```python
from build123d import *

# Parameters (mm, degrees)
F0_R      = 20
F1_DEPTH  = 47.5
F3_DEPTH  = 30
F5_DEPTH  = 25
F7_DEPTH  = 30
F8_R      = 6
F9_DEPTH  = 25
F10_DEPTH = 57.501


with BuildPart() as f1:
    # F0 (on Front) → F1 (new body, symmetric)
    with BuildSketch(Plane.XZ):
        Circle(F0_R)
    extrude(amount=F1_DEPTH, both=True)

    # F2 (on face) → F3 (cut)
    with BuildSketch(Plane.XZ.offset(47.5)):
        with BuildLine():
            ThreePointArc((8, 18.3303027798), (0, 20), (-8, 18.3303027798))
            Line((-8, 18.3303027798), (-8, -18.3303027798))
            ThreePointArc((-8, -18.3303027798), (0, -20), (8, -18.3303027798))
            Line((8, -18.3303027798), (8, 18.3303027798))
        make_face()
    extrude(amount=-F3_DEPTH, mode=Mode.SUBTRACT)

    # F4 (on face) → F5 (cut)
    with BuildSketch(Plane.XZ.offset(47.5)):
        with BuildLine():
            Line((-18, -8.7177978871), (-18, 8.7177978871))
            ThreePointArc((-18, 8.7177978871), (-20, 0), (-18, -8.7177978871))
        make_face()
        with BuildLine():
            ThreePointArc((20, 0), (19.4935886896, 4.472135955), (18, 8.7177978871))
            Line((18, 8.7177978871), (18, -8.7177978871))
            ThreePointArc((18, -8.7177978871), (19.4935886896, -4.472135955), (20, 0))
        make_face()
    extrude(amount=-F5_DEPTH, mode=Mode.SUBTRACT)

    # F6 (on face) → F7 (cut)
    with BuildSketch(Plane(origin=(0, 47.5, 0), x_dir=(-1, 0, 0), z_dir=(0, 1, 0))):
        with BuildLine():
            Line((-15.612494996, 12.5), (15.612494996, 12.5))
            ThreePointArc((15.612494996, 12.5), (0, 20), (-15.612494996, 12.5))
        make_face()
        with BuildLine():
            Line((15.612494996, -12.5), (-15.612494996, -12.5))
            ThreePointArc((-15.612494996, -12.5), (0, -20), (15.612494996, -12.5))
        make_face()
    extrude(amount=-F7_DEPTH, mode=Mode.SUBTRACT)

    # F8 (on face) → F9 (join)
    with BuildSketch(Plane.XY.offset(12.5)):
        with Locations((0, 31.5)):
            Circle(F8_R)
    extrude(amount=F9_DEPTH)

    # F10 (cut, through all): a face of the model
    f10_faces = [f1.faces().sort_by_distance(p)[0] for p in [
        (0, 31.5, 37.5),
    ]]
    extrude(f10_faces, amount=-F10_DEPTH, mode=Mode.SUBTRACT)


solid = f1.part
```
Check sheet for the modelled part. Datum: model origin and axes. Units: mm. A direction names the side the tool comes from. Round coordinates to 2 decimals unless told otherwise and drop trailing zeros. Order: outer loops, then holes, each group sorted by start corner. A loop starts at its lowest first (then second) coordinate and runs counter-clockwise, first axis right, second up. Notation, with made-up numbers: M -13.5,63 L 34.5,63 A28 ccw 34.5,87 Z; hole C 54.25,70 d3. An arc over 180 degrees is marked long. Answer in a Markdown table with one row per item.
(1) Set-up check for faces 1 (the flat face through (0, 39, -12.5)), 2 (the flat face through (8, -33, 0)), 3 (the flat face through (0, 17.5, 15)): record each of +Z, -Z, +X, -X, +Y, -Y from which the full face is reachable in a straight line by a thin tool's end or side.
Findings:
| item | result |
|---|---|
| face 1 | -Z, +X, -X, +Y |
| face 2 | +Z, -Z, -Y |
| face 3 | +Z, +X, -X, +Y |
(2) Section check D-D on z = -17. Record the boundary of the cut face in (x, y).
Findings:
| item | result |
|---|---|
| outline | M -10.54,-47.5 L -8,-47.5 L -8,-17.5 L 8,-17.5 L 8,-47.5 L 10.54,-47.5 L 10.54,17.5 L -10.54,17.5 Z |
(3) Draft check along X on faces 4 (the flat face through (-18, -35, 0)), 5 (the flat face through (-8, -33, 0)), 6 (the flat face through (0, 39, 12.5)). Enter one of: +X half, -X half, draft (parallel to the pull), parting line (faces both ways), or undercut.
Findings:
| item | result |
|---|---|
| face 4 | -X half |
| face 5 | undercut |
| face 6 | draft |
(4) Gauge pin test, flat ends, axial feed: pin 1 (3 mm diameter, centred on y = 22, z = 12.5, fed in from -X); pin 2 (6 mm diameter, centred on x = -2, z = 18, fed in from +Y); pin 3 (4 mm diameter, centred on x = -6, y = -14.5, fed in from +Z). Record the tip position at first contact, or that the pin passes through.
Findings:
| item | result |
|---|---|
| pin 1 | stops at x = -16.7 |
| pin 2 | stops at y = 17.5 |
| pin 3 | stops at z = 19.6 |
(5) Material ranges on line 1 along Y through (x, z) = (0, -2); line 2 along X through (y, z) = (-36.5, 5); line 3 along Z through (x, y) = (0.5, -10.5), recorded low to high. Write a range as from..to.
Findings:
| item | result |
|---|---|
| line 1 | y = -17.5..25.5, 37.5..47.5 |
| line 2 | x = -18..-8, 8..18 |
| line 3 | z = -19.99..19.99 |
(6) Section check C-C on z = 0. Record the boundary of the cut face in (x, y), plus the area to 3 significant figures.
Findings:
| item | result |
|---|---|
| outline | M -20,-22.5 L -18,-22.5 L -18,-47.5 L -8,-47.5 L -8,-17.5 L 8,-17.5 L 8,-47.5 L 18,-47.5 L 18,-22.5 L 20,-22.5 L 20,47.5 L -20,47.5 Z; hole C 0,31.5 d12 |
| area | 3,110 mm^2 |
(7) Section check B-B on x = 0. Record the boundary of the cut face in (y, z).
Findings:
| item | result |
|---|---|
| outline | M -17.5,-20 L 17.5,-20 L 17.5,-12.5 L 25.5,-12.5 L 25.5,12.5 L 17.5,12.5 L 17.5,20 L -17.5,20 Z; M 37.5,-12.5 L 47.5,-12.5 L 47.5,12.5 L 37.5,12.5 Z |
(8) Section check A-A on y = 31.5. Record the boundary of the cut face in (x, z), plus the area to 3 significant figures.
Findings:
| item | result |
|---|---|
| outline | M -15.61,-12.5 L -6,-12.5 L -6,12.5 L -15.61,12.5 A20 ccw Z; M 6,-12.5 L 15.61,-12.5 A20 ccw 15.61,12.5 L 6,12.5 Z |
| area | 630 mm^2 |
